from build123d import *

# Parameters (mm, degrees)
EXTRUDE_1_DEPTH     = 25
SKETCH_2_W          = 5
SKETCH_2_H          = 15
CUT_EXTRUDE_1_DEPTH = 309.879021625
SKETCH_3_R          = 5
CUT_EXTRUDE_2_DEPTH = 309.605735527


with BuildPart() as part:
    # 草图1 → 凸台-拉伸1 (new body)
    with BuildSketch(Plane.XY):
        with BuildLine():
            Line((-7.5, 0), (-7.5, 300))
            ThreePointArc((-7.5, 300), (0, 307.5), (7.5, 300))
            Line((7.5, 300), (7.5, 0))
            ThreePointArc((7.5, 0), (0, -7.5), (-7.5, 0))
        make_face()
    extrude(amount=EXTRUDE_1_DEPTH)

    # 草图2 → 切除-拉伸1 (cut, through all)
    with BuildSketch(Plane(origin=(7.5, 0, 0), x_dir=(0, 0, -1), z_dir=(1, 0, 0))):
        with Locations((-12.5, 300)):
            Rectangle(SKETCH_2_W, SKETCH_2_H)
        with Locations((-12.5, 0)):
            Rectangle(SKETCH_2_W, SKETCH_2_H)
    extrude(amount=-CUT_EXTRUDE_1_DEPTH, mode=Mode.SUBTRACT)

    # 草图3 → 切除-拉伸2 (cut, through all)
    with BuildSketch(Plane.XY.offset(25)):
        with Locations((0, 300)):
            Circle(SKETCH_3_R)
        Circle(SKETCH_3_R)
    extrude(amount=-CUT_EXTRUDE_2_DEPTH, mode=Mode.SUBTRACT)


solid = part.part
Design review of the part built by this model. Coordinates are the model's own, in mm. A direction names the side the tool comes from. Round coordinates to 2 decimals unless told otherwise and drop trailing zeros. Order: outer loops, then holes, each group sorted by start corner. A loop starts at its lowest first (then second) coordinate and runs counter-clockwise, first axis right, second up.
1) Machinability: for faces 1 (the flat face through (-2, 295, 10)), 2 (the cylindrical face through (-0.651, 304.957, 5.07)), 3 (the flat face through (-2, 5, 10)), which of the approach directions +Z, -Z, +X, -X, +Y, -Y give a long, thin tool a straight path to every point of the face, cutting with its end or side? Answer none if there is none.
The answers:
face 1: +X, -X, +Y
face 2: +Z, -Z
face 3: +X, -X, -Y
2) Clearance check with flat-ended pins moving along their axes: pin 1 Ø5.5 at (x, z) = (3, 13) entering from +Y; pin 2 Ø3 at (x, z) = (-2.5, 19) entering from -Y; pin 3 Ø1.5 at (x, z) = (-3.5, 13) entering from -Y. State where each tip first meets the part, or that it passes through.
The answers:
pin 1: stops at y = 307.42
pin 2: stops at y = -7.43
pin 3: stops at y = 7.5
3) Consider section A-A (x = 0). State the section outline as (y, z) points.
The answers:
outline: (-7.5, 0) - (-5, 0) - (-5, 10) - (-7.5, 10) - close; (-7.5, 15) - (-5, 15) - (-5, 25) - (-7.5, 25) - close; (5, 0) - (295, 0) - (295, 10) - (292.5, 10) - (292.5, 15) - (295, 15) - (295, 25) - (5, 25) - (5, 15) - (7.5, 15) - (7.5, 10) - (5, 10) - close; (305, 0) - (307.5, 0) - (307.5, 10) - (305, 10) - close; (305, 15) - (307.5, 15) - (307.5, 25) - (305, 25) - close
4) Consider section B-B (z = 5). State the section outline as (x, y) points, plus the area to 3 significant figures.
The answers:
outline: (-7.5, 0) arc R7.5 ccw to (7.5, 0) - (7.5, 300) arc R7.5 ccw to (-7.5, 300) - close; hole circle Ø10 at (0, 0); hole circle Ø10 at (0, 300)
area: 4,520 mm2
5) Draft analysis for pull direction X (two halves, no side actions). For faces 4 (the cylindrical face through (-1.08, -4.88, 5.07)), 5 (the cylindrical face through (-0.651, 304.957, 20.07)), 6 (the flat face through (-7.5, 148, 12)), 7 (the cylindrical face through (-0.16, 307.5, 19.93)), state which applies: released by +X, released by -X, zero draft, split by the parting line, or undercut.
The answers:
face 4: undercut
face 5: undercut
face 6: released by -X
face 7: split by the parting line
6) For L1, parallel to Y at x = -0.5, z = 23.5; L2, parallel to X at y = 300, z = 20.25; L3, parallel to Y at x = -3.5, z = 2.75, list the stretches that pass through material, from the lowest coordinate up.
The answers:
L1: y = -7.48 to -4.97, 4.97 to 295.03, 304.97 to 307.48
L2: x = -7.5 to -5, 5 to 7.5
L3: y = -6.63 to -3.57, 3.57 to 296.43, 303.57 to 306.63
